```python
from build123d import *

# Parameters (mm, degrees)
F1_DEPTH = 2
F3_DEPTH = 5


with BuildPart() as f1:
    # F0 (on Top) → F1 (new body)
    with BuildSketch(Plane.XY):
        Polygon((0, 164.685234), (-86.34713, 15), (-69.030312, 15), (-37.203411, 70.172849), (0, 134.666033), (37.203411, 70.172849), (69.030312, 15), (86.34713, 15), align=None)
        Polygon((-89.227728, 0), (0, 0), (89.227728, 0), (86.343437, 5), (92.11571, 5), (86.34713, 15), (69.030312, 15), (0, 15), (-69.030312, 15), (-86.34713, 15), (-95, 0), align=None)
        Polygon((86.343437, 5), (89.227728, 0), (95, 0), (92.11571, 5), align=None)
        Polygon((-37.203411, 70.172849), (-69.030312, 15), (0, 15), (69.030312, 15), (37.203411, 70.172849), (0, 134.666033), align=None)
    extrude(amount=F1_DEPTH)

    # F2 (on face) → F3 (join)
    with BuildSketch(Plane(origin=(0, 0, 0), x_dir=(1, 0, 0), z_dir=(0, 0, -1))):
        Polygon((1.73242, -150.674994), (52.60681, -62.482775), (50.87439, -61.483415), (0, -149.675634), (-50.87439, -61.483415), (-82.015156, -7.5), (-83.168872, -5.5), (-85.477781, -5.5), (-1.73242, -150.674994), align=None)
        Polygon((0, -7.5), (82.015156, -7.5), (83.168872, -5.5), (-12.322525, -5.5), (-83.168872, -5.5), (-82.015156, -7.5), align=None)
        Polygon((50.87439, -61.483415), (52.60681, -62.482775), (85.477781, -5.5), (83.168872, -5.5), (82.015156, -7.5), align=None)
    extrude(amount=F3_DEPTH)


solid = f1.part
```
Can you work these out from the model? Positions are in its coordinate system, mm. A direction names the side the tool comes from. Give positions to 0.01 mm unless a question says otherwise; leave off trailing zeros. Order: outer loops, then holes, each group sorted by start corner. A loop starts at its lowest first (then second) coordinate and runs counter-clockwise, first axis right, second up. Notation, with made-up numbers: M 49,35.5 L 70,35.5 A16 cw 70,48.5 Z; hole C 42,25 d5. An arc over 180 degrees is marked long. Write item = value, one per line. Start each with the question number.
Q1. I need wall thicknesses on probe 1 along Z at (x, y) = (-61, 19.5); probe 2 along Y at (x, z) = (38.5, -3.25); probe 3 along X at (y, z) = (110.5, -1.75). Which ranges of each line are inside material? Lowest first, please. Write a range as [from, to].
Q2. Suppose I cut it at A-A (z = -2.25). Write out the boundary of the cut face in (x, y) (3 decimals).
Q3. Will these pins go through, and if not, where does the flat tip stop? pin 1 Ø1.5 at (x, z) = (5, -2) entering from +Y; pin 2 Ø4 at (x, z) = (-0.5, -2.5) entering from +Y (3 decimals); pin 3 Ø1 at (y, z) = (83.5, -2) entering from +X.
Q4. For faces 4 (the flat face through (1, 5.5, -2)), 5 (the flat face through (-45, 72, -5)), 6 (the flat face through (-1, 64, 0)), which set-ups out of +Z, -Z, +X, -X, +Y, -Y let a thin tool reach every point of the face, with its end or its side?
Q5. Suppose I cut it at C-C (y = 38.5). Write out the boundary of the cut face in (x, z).
Q6. Suppose I cut it at B-B (x = 32.5). Write out the boundary of the cut face in (y, z).
Q7. We'd pull the mould along X, two halves only. Please class faces 1 (the flat face through (-44.19, 77.07, -2.46)), 2 (the flat face through (-1, 7.5, -2)), 3 (the flat face through (-1, 65, 2)): pulls with the +X half, pulls with the -X half, needs draft (parallel to the pull), parting line crosses it, or undercut.
Q8. Suppose I cut it at D-D (y = 153.5). Write out the boundary of the cut face in (x, z), plus the area to 3 significant figures.
Check result:
q1.probe_1 = [0, 2]
q1.probe_2 = [5.5, 7.5], [82.93, 86.94]
q1.probe_3 = [-24.91, -22.6], [22.6, 24.91]
q2.outline = M -85.478,5.5 L 85.478,5.5 L 1.732,150.675 L -1.732,150.675 Z; hole M -82.015,7.5 L 82.015,7.5 L 0,149.676 Z
q3.pin_1 = 146.31
q3.pin_2 = 150.675
q3.pin_3 = 40.77
q4.face_4 = -Z, +X, -X, -Y
q4.face_5 = -Z, +X, -X, +Y, -Y
q4.face_6 = -Z
q5.outline = M -72.79,0 L -66.44,0 L -66.44,-5 L -64.13,-5 L -64.13,0 L 64.13,0 L 64.13,-5 L 66.44,-5 L 66.44,0 L 72.79,0 L 72.79,2 L -72.79,2 Z
q6.outline = M 0,0 L 5.5,0 L 5.5,-5 L 7.5,-5 L 7.5,0 L 93.34,0 L 93.34,-5 L 97.34,-5 L 97.34,0 L 108.35,0 L 108.35,2 L 0,2 Z
q7.face_1 = pulls with the -X half
q7.face_2 = undercut
q7.face_3 = needs draft
q8.outline = M -6.45,0 L 6.45,0 L 6.45,2 L -6.45,2 Z
q8.area = 25.8 mm2
